Input: part model. Units: mm. Frame: model coordinates. Round coordinates to 2 decimals unless told otherwise and drop trailing zeros. Loops run counter-clockwise (first coordinate to the right, second up) from the corner with the lowest first, then second, coordinate; pieces in that order, holes last. Notation, with made-up numbers: (61.5, 72.25) -> (92.5, 72.25) arc R25 cw to (92.5, 93.25) -> close; hole circle Ø7 at (-20, 71). An arc over 180 degrees is marked (long way). One line per question, with ' | ' between items. Start each with the question number.
Q1. Cut plane B-B on y = 3.35. State how many separate pieces and enclosed holes the cut face has, and give its area (3 significant figures).
Q2. Cut plane A-A on z = -158.4. Return loops of the section in (x, y).
Q3. Material intervals for L1, parallel to X at y = 1.7, z = -170; L2, parallel to X at y = 2.95, z = -60; L3, parallel to X at y = 2.5, z = -10, sorted ascending.
Q4. Mould query, pull axis Z, two halves, no side actions, for faces 1 (the face through (-206.33, 3.042, -149.163)), 2 (the face through (3, 0, -91)), 3 (the face through (198.67, 3.042, -149.163)). Classes: pulls with the +Z half, pulls with the -Z half, needs draft (parallel to the pull), parting line crosses it, or undercut.
Q5. Contact query for a flat-ended pin moving along its axis: P1, Ø6.5, axis at x = -222.5, z = -60, coming from the +Y side. Output: stop coordinate, or through.
from build123d import *

# Parameters (mm, degrees)
BOSS_EXTRUDE1_DEPTH = 6
SKETCH2_R           = 2.5
CUT_EXTRUDE1_DEPTH  = 295.095647707
FILLET1_R           = 4
SKETCH3_R           = 10
CUT_EXTRUDE2_DEPTH  = 295.095647707


with BuildPart() as part:
    # Sketch1 → Boss-Extrude1 (new body)
    with BuildSketch(Plane(origin=(0, 0, 0), x_dir=(1, 0, 0), z_dir=(0, 1, 0))):
        Polygon((0, 0), (-182.5, 0), (-182.5, 50), (-232.5, 50), (-232.5, 180), (232.5, 180), (232.5, 50), (182.5, 50), (182.5, 0), align=None)
    extrude(amount=BOSS_EXTRUDE1_DEPTH)

    # Sketch2 → Cut-Extrude1 (cut, through all)
    with BuildSketch(Plane(origin=(0, 6, 0), x_dir=(1, 0, 0), z_dir=(0, 1, 0))):
        with Locations(Location((-222.5, 170, 0), (0, 0, 270))):
            Circle(SKETCH2_R)
        with Locations(Location((-222.5, 60, 0), (0, 0, 270))):
            Circle(SKETCH2_R)
        with Locations(Location((222.5, 170, 0), (0, 0, 270))):
            Circle(SKETCH2_R)
        with Locations(Location((222.5, 60, 0), (0, 0, 270))):
            Circle(SKETCH2_R)
        with Locations(Location((-172.5, 10, 0), (0, 0, 270))):
            Circle(SKETCH2_R)
        with Locations(Location((-86.25, 10, 0), (0, 0, 270))):
            Circle(SKETCH2_R)
        with Locations(Location((0, 10, 0), (0, 0, 270))):
            Circle(SKETCH2_R)
        with Locations(Location((86.25, 10, 0), (0, 0, 270))):
            Circle(SKETCH2_R)
        with Locations(Location((172.5, 10, 0), (0, 0, 270))):
            Circle(SKETCH2_R)
        with Locations(Location((-162.5, 170, 0), (0, 0, 270))):
            Circle(SKETCH2_R)
        with Locations(Location((162.5, 170, 0), (0, 0, 270))):
            Circle(SKETCH2_R)
    extrude(amount=-CUT_EXTRUDE1_DEPTH, mode=Mode.SUBTRACT)

    # Fillet1
    fillet1_edges = [part.edges().sort_by_distance(p)[0] for p in [
        (-182.5, 3, -50),
        (182.5, 3, -50),
    ]]
    fillet(fillet1_edges, radius=FILLET1_R)

    # Sketch3 → Cut-Extrude2 (cut, through all)
    with BuildSketch(Plane(origin=(0, 6, 0), x_dir=(1, 0, 0), z_dir=(0, 1, 0))):
        with Locations(Location((-202.5, 158.4, 0), (0, 0, 270))):
            Circle(SKETCH3_R)
        with Locations(Location((202.5, 158.4, 0), (0, 0, 270))):
            Circle(SKETCH3_R)
    extrude(amount=-CUT_EXTRUDE2_DEPTH, mode=Mode.SUBTRACT)


solid = part.part
Results:
1) separate pieces: 1 | enclosed holes: 13 | area: 77,900 mm^2
2) outline: (-232.5, 0) -> (-212.5, 0) -> (-212.5, 6) -> (-232.5, 6) -> close; (-192.5, 0) -> (192.5, 0) -> (192.5, 6) -> (-192.5, 6) -> close; (212.5, 0) -> (232.5, 0) -> (232.5, 6) -> (212.5, 6) -> close
3) L1: -232.5 to -225, -220 to -165, -160 to 160, 165 to 220, 225 to 232.5 | L2: -232.5 to -225, -220 to 220, 225 to 232.5 | L3: -182.5 to -175, -170 to -88.75, -83.75 to -2.5, 2.5 to 83.75, 88.75 to 170, 175 to 182.5
4) face 1: undercut | face 2: needs draft | face 3: undercut
5) P1: y = 6
